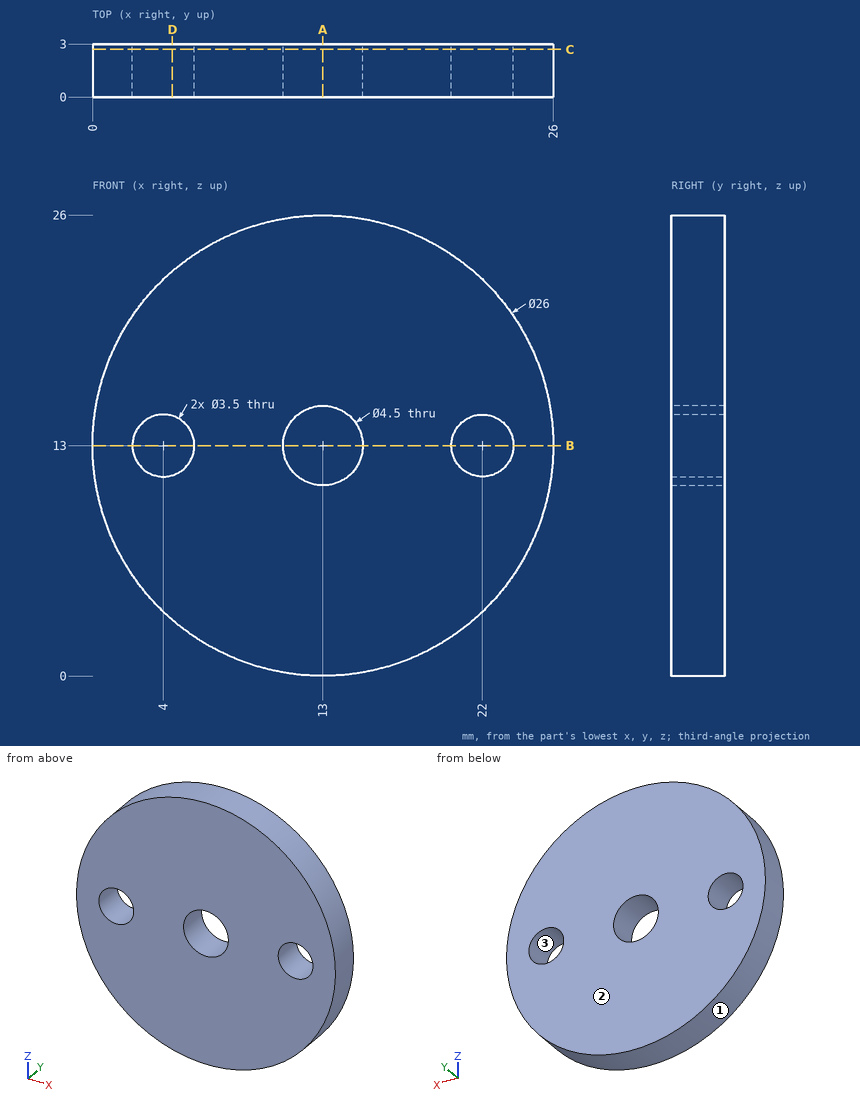
Check sheet for the drawn part. Datum: minimum x, y, z corner. Units: mm. Round coordinates to 2 decimals unless told otherwise and drop trailing zeros. Loops run counter-clockwise (first coordinate to the right, second up) from the corner with the lowest first, then second, coordinate; pieces in that order, holes last. Notation, with made-up numbers: (28.25, 45) - (36.25, 45) arc R33 cw to (36.25, 76) - close; hole circle Ø11 at (73, -12). An arc over 180 degrees is marked (long way). Write each question's results on one line, items separated by ' | '. Start each with the question number.
Q1. Thickness scan on line 1 (X direction, y = 1.35, z = 13); line 2 (Z direction, x = 23, y = 0.1); line 3 (Z direction, x = 4.5, y = 1). Record the ranges inside material, lowest first. Write a range as [from, to].
Q2. Cross-section at D-D on x = 4.5. Enter the section's corners in (y, z).
Q3. Release check for a two-part mould opening along X. For the marked faces 1, 2 and 3 record: +X half, -X half, draft (parallel to the pull), parting line (faces both ways), or undercut.
Q4. Cross-section at A-A on x = 13. Enter the section's corners in (y, z), and give its area (3 significant figures).
Q5. Gauge pin test, flat ends, axial feed: P1, Ø3, axis at x = 22, z = 13, coming from the +Y side; P2, Ø1.5, axis at x = 4.5, y = 2, coming from the +Z side. Record the tip position at first contact, or that the pin passes through.
Q6. Cross-section at B-B on z = 13. Enter the section's corners in (x, y), and give its area (3 significant figures).
Q7. Cross-section at C-C on y = 2.7. Enter the section's corners in (x, z).
Answers below:
1) line 1: x = [0, 2.25], [5.75, 10.75], [15.25, 20.25], [23.75, 26] | line 2: z = [4.69, 11.56], [14.44, 21.31] | line 3: z = [3.16, 11.32], [14.68, 22.84]
2) outline: (0, 3.16) - (3, 3.16) - (3, 11.32) - (0, 11.32) - close; (0, 14.68) - (3, 14.68) - (3, 22.84) - (0, 22.84) - close
3) face 1: parting line | face 2: draft | face 3: undercut
4) outline: (0, 0) - (3, 0) - (3, 10.75) - (0, 10.75) - close; (0, 15.25) - (3, 15.25) - (3, 26) - (0, 26) - close | area: 64.5 mm²
5) P1: passes through | P2: stops at z = 23.44
6) outline: (0, 0) - (2.25, 0) - (2.25, 3) - (0, 3) - close; (5.75, 0) - (10.75, 0) - (10.75, 3) - (5.75, 3) - close; (15.25, 0) - (20.25, 0) - (20.25, 3) - (15.25, 3) - close; (23.75, 0) - (26, 0) - (26, 3) - (23.75, 3) - close | area: 43.5 mm²
7) outline: circle Ø26 at (13, 13); hole circle Ø3.5 at (4, 13); hole circle Ø4.5 at (13, 13); hole circle Ø3.5 at (22, 13)
